```python
from build123d import *

# Parameters (mm, degrees)
SKETCH1_W           = 17.78
SKETCH1_H           = 16.002
SKETCH1_W_2         = 12.7
SKETCH1_H_2         = 6.858
BOSS_EXTRUDE1_DEPTH = 2.54
SKETCH2_R           = 1.44
CUT_EXTRUDE1_DEPTH  = 24.164535415
SKETCH3_W           = 12.7
SKETCH3_H           = 2.54
BOSS_EXTRUDE2_DEPTH = 10.16
SKETCH4_W           = 17.78
SKETCH4_H           = 16.002
BOSS_EXTRUDE3_DEPTH = 2.54
SKETCH5_R           = 2
SKETCH5_R_2         = 0.8
CUT_EXTRUDE2_DEPTH  = 30.723426855


with BuildPart() as part:
    # Sketch1 → Boss-Extrude1 (new body)
    with BuildSketch(Plane(origin=(0, 0, 0), x_dir=(1, 0, 0), z_dir=(0, 1, 0))):
        Rectangle(SKETCH1_W, SKETCH1_H)
        with Locations((-15.24, 0)):
            Rectangle(SKETCH1_W_2, SKETCH1_H_2)
        with Locations((15.24, 0)):
            Rectangle(SKETCH1_W_2, SKETCH1_H_2)
    extrude(amount=BOSS_EXTRUDE1_DEPTH)

    # Sketch2 → Cut-Extrude1 (cut, through all)
    with BuildSketch(Plane.XZ):
        with Locations(Location((-17.78, 0, 0), (0, 0, 270))):
            Circle(SKETCH2_R)
        with Locations(Location((17.78, 0, 0), (0, 0, 270))):
            Circle(SKETCH2_R)
    extrude(amount=-CUT_EXTRUDE1_DEPTH, mode=Mode.SUBTRACT)

    # Sketch3 → Boss-Extrude2 (add)
    with BuildSketch(Plane(origin=(0, 0, 0), x_dir=(-1, 0, 0), z_dir=(0, -1, 0))):
        Polygon((6.35, -8.001), (8.89, -8.001), (8.89, -3.429), (8.89, 3.429), (8.89, 8.001), (6.35, 8.001), (6.35, 5.461), align=None)
        with Locations((0, 6.731)):
            Rectangle(SKETCH3_W, SKETCH3_H)
        Polygon((-8.89, -8.001), (-6.35, -8.001), (-6.35, 5.461), (-6.35, 8.001), (-8.89, 8.001), (-8.89, 3.429), (-8.89, -3.429), align=None)
    extrude(amount=BOSS_EXTRUDE2_DEPTH)

    # Sketch4 → Boss-Extrude3 (add)
    with BuildSketch(Plane(origin=(0, -10.16, 0), x_dir=(-1, 0, 0), z_dir=(0, -1, 0))):
        Rectangle(SKETCH4_W, SKETCH4_H)
    extrude(amount=BOSS_EXTRUDE3_DEPTH)

    # Sketch5 → Cut-Extrude2 (cut, through all)
    with BuildSketch(Plane(origin=(0, 0, -8.001), x_dir=(-1, 0, 0), z_dir=(0, 0, -1))):
        with Locations((0, -5.08)):
            Circle(SKETCH5_R)
        with Locations((4.699, -5.08)):
            Circle(SKETCH5_R_2)
        with Locations((-4.699, -5.08)):
            Circle(SKETCH5_R_2)
    extrude(amount=-CUT_EXTRUDE2_DEPTH, mode=Mode.SUBTRACT)


solid = part.part
```
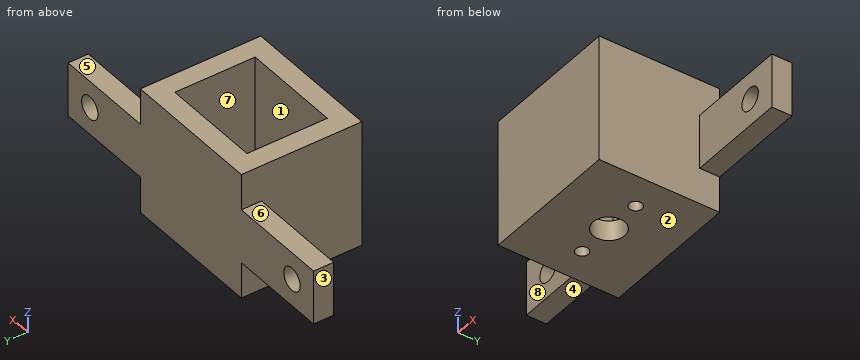
Here's how the part is built. I have some questions about the finished solid (model axes, mm). Face numbers are marked on the shaded views. A direction names the side the tool comes from. Coordinates: 2 decimals unless noted, no trailing zeros. Order: outer loops, then holes, each group sorted by start corner. A loop starts at its lowest first (then second) coordinate and runs counter-clockwise, first axis right, second up.
1) Which directions (+Z, -Z, +X, -X, +Y, -Y) give clear straight access to the entire face, cutting with the end or side of a thin tool? Please do the marked faces 4, 5, 6, 7 and 8.
2) I need wall thicknesses on line 1 (X direction, y = 1.75, z = 0); line 2 (X direction, y = -5, z = -4.5); line 3 (Y direction, x = 0, z = -7.4). Which ranges of each line are inside material? Lowest first, please.
3) We'd pull the mould along X, two halves only. Please class the marked faces 1, 2 and 3: +X half, -X half, draft (parallel to the pull), parting line (faces both ways), or undercut.
4) Will these pins go through, and if not, where does the flat tip stop? pin 1 (2 mm diameter, centred on x = -17.5, y = 1.5, fed in from +Z); pin 2 (5.5 mm diameter, centred on x = -18.5, z = 1, fed in from -Y); pin 3 (6.5 mm diameter, centred on x = 0, y = -5.08, fed in from +Z).
5) Imagine slicing it at C-C on z = 0. List the corners of the cut face in (x, y) for me.
6) Imagine slicing it at A-A on x = -17.78. List the corners of the cut face in (y, z) for me.
7) Imagine slicing it at D-D on y = -5.08. List the corners of the cut face in (x, z) for me, and give its area (3 significant figures).
8) Imagine slicing it at B-B on z = 6.75. List the corners of the cut face in (x, y) for me, and give its area (3 significant figures).
Response values:
1. face 4: -Z, -X, +Y, -Y
1. face 5: +Z, +X, +Y, -Y
1. face 6: +Z, -X, +Y, -Y
1. face 7: +Z
1. face 8: +Z, -Z, -X, -Y
2. line 1: x = -21.59 to -19.22, -16.34 to 16.34, 19.22 to 21.59
2. line 2: x = -8.89 to -6.35, 6.35 to 8.89
2. line 3: y = -12.7 to -7.08, -3.08 to 2.54
3. face 1: undercut
3. face 2: draft
3. face 3: -X half
4. pin 1: stops at z = 3.43
4. pin 2: stops at y = 0
4. pin 3: stops at z = -5.46
5. outline: (-21.59, 0) - (-19.22, 0) - (-19.22, 2.54) - (-21.59, 2.54) - close; (-16.34, 0) - (-8.89, 0) - (-8.89, -12.7) - (8.89, -12.7) - (8.89, 0) - (16.34, 0) - (16.34, 2.54) - (-16.34, 2.54) - close; (19.22, 0) - (21.59, 0) - (21.59, 2.54) - (19.22, 2.54) - close; hole (-6.35, -10.16) - (6.35, -10.16) - (6.35, 0) - (-6.35, 0) - close
6. outline: (0, -3.43) - (2.54, -3.43) - (2.54, -1.44) - (0, -1.44) - close; (0, 1.44) - (2.54, 1.44) - (2.54, 3.43) - (0, 3.43) - close
7. outline: (-8.89, -8) - (-5.5, -8) - (-5.5, -5.46) - (-6.35, -5.46) - (-6.35, 8) - (-8.89, 8) - close; (-3.9, -8) - (-2, -8) - (-2, -5.46) - (-3.9, -5.46) - close; (2, -8) - (3.9, -8) - (3.9, -5.46) - (2, -5.46) - close; (5.5, -8) - (8.89, -8) - (8.89, 8) - (6.35, 8) - (6.35, -5.46) - (5.5, -5.46) - close
7. area: 95.3 mm2
8. outline: (-8.89, -12.7) - (8.89, -12.7) - (8.89, 2.54) - (-8.89, 2.54) - close; hole (-6.35, -10.16) - (6.35, -10.16) - (6.35, 0) - (-6.35, 0) - close
8. area: 142 mm2
